Can you work these out from the model? Positions are in its coordinate system, mm. Face numbers are marked on the shaded views. Give positions to 0.01 mm unless a question says otherwise; leave off trailing zeros. Order: outer loops, then holes, each group sorted by start corner. A loop starts at its lowest first (then second) coordinate and runs counter-clockwise, first axis right, second up. Notation, with made-up numbers: M 60.25,0 L 98.25,0 A24 cw 98.25,21 Z; hole C 23,2.5 d6. An arc over 180 degrees is marked long. Use one line per item in the form item = value. Start each with the question number.
1. I want a section at C-C, the plane y = 33.5. List the corners of the cut face in (x, z) for me.
2. I want a section at A-A, the plane z = 0. Count the separate pieces of the cut face and the enclosed holes in it, and give its area (3 significant figures).
3. Will these pins go through, and if not, where does the flat tip stop? P1, Ø6, axis at y = 7, z = -1.5, coming from the +X side; P2, Ø2, axis at x = -7.5, z = 17, coming from the -Y side; P3, Ø1, axis at y = 26, z = -12, coming from the +X side.
4. I need wall thicknesses on L1, parallel to X at y = 20, z = 0; L2, parallel to Z at x = 45, y = 30; L3, parallel to Y at x = 54.5, z = -10.5. Which ranges of each line are inside material? Lowest first, please.
5. We'd pull the mould along X, two halves only. Please class the marked faces 1, 2, 3 and 4: +X half, -X half, draft (parallel to the pull), parting line (faces both ways), or undercut.
6. I want a section at B-B, the plane x = 50. List the corners of the cut face in (y, z) for me.
```python
from build123d import *

# Parameters (mm, degrees)
SKETCH1_R           = 19.2
BOSS_EXTRUDE1_DEPTH = 40
SHELL1_T            = -6
CHAMFER1_SIZE       = 1
RIB1_REACH          = 118.241
SKETCH2_WALLS_W     = 6
SKETCH2_WALLS_H     = 263.960304727
FILLET1_R           = 1
BOSS_EXTRUDE2_START = -3
BOSS_EXTRUDE2_DEPTH = 3
CHAMFER2_SIZE       = 0.5


with BuildPart() as part:
    # Sketch1 → Boss-Extrude1 (new body)
    with BuildSketch(Plane(origin=(0, 0, 0), x_dir=(1, 0, 0), z_dir=(0, 1, 0))):
        with BuildLine():
            Line((0, 26), (80, 26))
            ThreePointArc((80, 26), (106, 0), (80, -26))
            Line((80, -26), (0, -26))
            ThreePointArc((0, -26), (-26, 0), (0, 26))
        make_face()
        with Locations(Location((0, 0, 0), (0, 0, 270))):
            Circle(SKETCH1_R, mode=Mode.SUBTRACT)
        with Locations(Location((80, 0, 0), (0, 0, 270))):
            Circle(SKETCH1_R, mode=Mode.SUBTRACT)
    extrude(amount=BOSS_EXTRUDE1_DEPTH)

    # Shell1
    shell1_openings = [part.faces().sort_by_distance(p)[0] for p in [
        (40, 40, 0),
    ]]
    offset(amount=SHELL1_T, openings=shell1_openings, kind=Kind.INTERSECTION)

    # Chamfer1
    chamfer1_edges = [part.edges().sort_by_distance(p)[0] for p in [
        (106, 40, 0),
        (40, 40, -26),
        (-26, 40, 0),
        (40, 0, -26),
        (106, 0, 0),
        (40, 0, 26),
        (-26, 0, 0),
        (40, 40, 26),
    ]]
    chamfer(chamfer1_edges, length=CHAMFER1_SIZE)

    # Sketch2 walls → Rib1 (add, up to next)
    with BuildSketch(Plane(origin=(0, 40, 0), x_dir=(1, 0, 0), z_dir=(0, 1, 0)), mode=Mode.PRIVATE) as rib1_sk1:
        with Locations((40, 0.813044615)):
            Rectangle(SKETCH2_WALLS_W, SKETCH2_WALLS_H)
    rib1_tool1 = extrude(rib1_sk1.sketch, amount=-RIB1_REACH, mode=Mode.PRIVATE) - part.part
    add(rib1_tool1.solids().sort_by_distance((40, 40, -0.813044614))[0])

    # Fillet1
    fillet1_edges = [part.edges().sort_by_distance(p)[0] for p in [
        (64.668985683, 23, 20),
        (15.331014317, 23, -20),
        (15.331014317, 23, 20),
        (64.668985683, 23, -20),
        (37, 23, 20),
        (37, 23, -20),
    ]]
    fillet(fillet1_edges, radius=FILLET1_R)

    # Sketch3 → Boss-Extrude2 (add)
    with BuildSketch(Plane(origin=(0, 40, 0), x_dir=(1, 0, 0), z_dir=(0, 1, 0)).offset(BOSS_EXTRUDE2_START)):
        with BuildLine():
            Line((18.039955654, 20), (61.960044346, 20))
            ThreePointArc((61.960044346, 20), (62.888804498, 19.370681238), (62.648592272, 18.27480916))
            ThreePointArc((62.648592272, 18.27480916), (54.8, 0), (62.648592272, -18.27480916))
            ThreePointArc((62.648592272, -18.27480916), (62.888804498, -19.370681238), (61.960044346, -20))
            Line((61.960044346, -20), (18.039955654, -20))
            ThreePointArc((18.039955654, -20), (17.111195502, -19.370681238), (17.351407728, -18.27480916))
            ThreePointArc((17.351407728, -18.27480916), (25.2, 0), (17.351407728, 18.27480916))
            ThreePointArc((17.351407728, 18.27480916), (17.111195502, 19.370681238), (18.039955654, 20))
        make_face()
    extrude(amount=BOSS_EXTRUDE2_DEPTH)

    # Chamfer2
    chamfer2_edges = [part.edges().sort_by_distance(p)[0] for p in [
        (0, 0, -19.2),
        (0, 40, -19.2),
        (80, 0, -19.2),
        (80, 40, -19.2),
    ]]
    chamfer(chamfer2_edges, length=CHAMFER2_SIZE)


solid = part.part
```
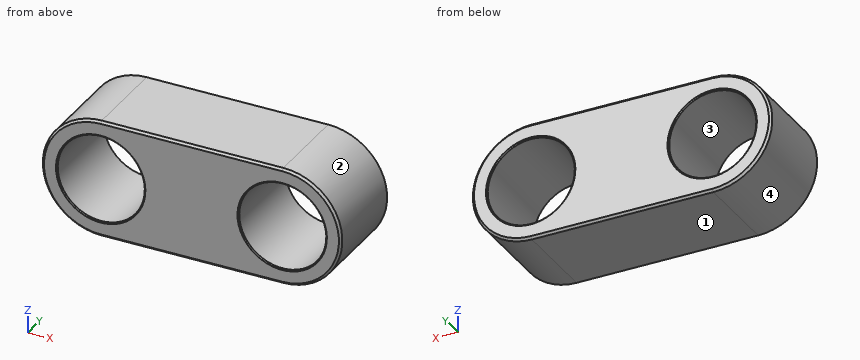
Check result:
q1.outline = M 0,-26 L 80,-26 A26 ccw 80,26 L 0,26 A26 ccw Z; hole C 0,0 d38.4; hole M 17.35,-18.27 A1 ccw 18.04,-20 L 36,-20 A1 ccw 37,-19 L 37,19 A1 ccw 36,20 L 18.04,20 A1 ccw 17.35,18.27 A25.2 cw Z; hole M 43,-20 L 61.96,-20 A1 ccw 62.65,-18.27 A25.2 cw 62.65,18.27 A1 ccw 61.96,20 L 43,20 Z; hole C 80,0 d38.4
q2.separate_pieces = 3
q2.enclosed_holes = 2
q2.area = 1,470 mm2
q3.P1 = 106
q3.P2 = 0.12
q3.P3 = 103.32
q4.L1 = -26 to -19.2, 19.2 to 25.2, 37 to 43, 54.8 to 60.8, 99.2 to 106
q4.L2 = -26 to -20, 20 to 26
q4.L3 = 0 to 6, 37 to 40
q5.face_1 = draft
q5.face_2 = +X half
q5.face_3 = undercut
q5.face_4 = -X half
q6.outline = M 0,-25 L 1,-26 L 39,-26 L 40,-25 L 40,25 L 39,26 L 1,26 L 0,25 Z; hole M 6,-20 L 37,-20 L 37,20 L 6,20 Z
